Geometry check sheet. Reference: the model listing, model coordinates, mm. Face numbers are marked on the shaded views. A direction names the side the tool comes from. Coordinates: 2 decimals unless noted, no trailing zeros. Order: outer loops, then holes, each group sorted by start corner. A loop starts at its lowest first (then second) coordinate and runs counter-clockwise, first axis right, second up.
Autodesk Inventor part; units mm, degrees
ref_plane "YZ Plane" through (0, 0, 0) normal (1, 0, 0) x (0, 1, 0)
ref_plane "XZ Plane" through (0, 0, 0) normal (0, 1, 0) x (-1, 0, 0)
ref_plane "XY Plane" through (0, 0, 0) normal (0, 0, 1) x (1, 0, 0)
sketch "Skizze1" plane through (0, 0, 0) normal (0, 1, 0) x (-1, 0, 0)
  circle A0 centre (0, 0) radius 3.5
  dimension "d0" = 7
extrude "Extrusion1" add sketch "Skizze1" along normal blind 13
sketch "Skizze2" plane through (0, 13, 0) normal (0, 1, 0) x (1, 0, 0)
  circle A0 centre (0, 0) radius 2.5
  dimension "d3" = 5
extrude "Extrusion2" cut sketch "Skizze2" against normal blind 0.35
sketch "Skizze3" plane through (0, 12.65, 0) normal (0, 1, 0) x (1, 0, 0)
  line L0 (0, 0) -> (0, 2.5) construction
  circle A0 centre (0, 0) radius 2.5 construction
  circle A1 centre (-1.27, 0) radius 0.75
  circle A2 centre (1.27, 0) radius 0.75
  dimension "d6" = 1.5
  dimension "d7" = 2.54
extrude "Extrusion3" cut sketch "Skizze3" against normal through all
properties part number "Abstandhalter_13mm" material "PC/ABS-Kunststoff"
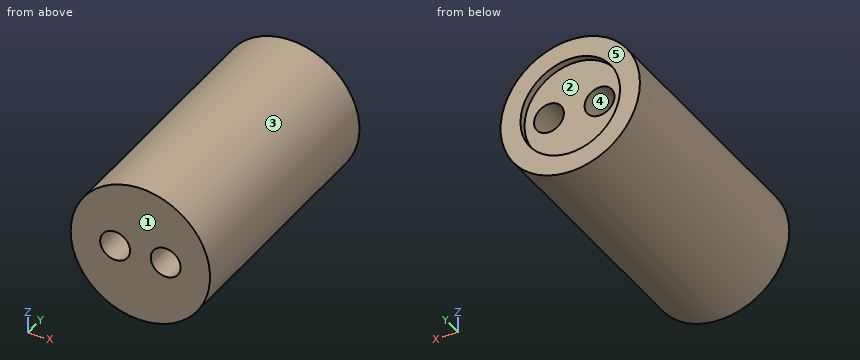
Item 1: Sectioned sample at A-A (z = 0). Record the cut outline in (x, y), and give its area (3 significant figures).
Item 2: Release check for a two-part mould opening along Z. For the marked faces 3, 4 and 5 record: pulls with the +Z half, pulls with the -Z half, needs draft (parallel to the pull), parting line crosses it, or undercut.
Item 3: Sectioned sample at C-C (x = 0.75). Record the cut outline in (y, z).
Item 4: Sectioned sample at D-D (y = 7.5). Record the cut outline in (x, z), and give its area (3 significant figures).
Item 5: Depth check by flat-ended pin: P1, Ø3, axis at x = 2, y = 3, coming from the +Z side; P2, Ø1, axis at x = -1, z = -0.5, coming from the -Y side; P3, Ø1.2, axis at x = 1.27, z = 0, coming from the +Y side; P4, Ø1.5, axis at y = 4.5, z = 2.5, coming from the +X side. Enter the tip coordinate at first touch or a pass-through.
Item 6: Sectioned sample at B-B (x = 0). Record the cut outline in (y, z), and give its area (4 significant figures).
Item 7: Tool access check on the marked faces 1 and 2. Record the directions out of +Z, -Z, +X, -X, +Y, -Y that give a thin tool (end or side, any length) a straight path to the whole face; none if there is none.
Item 8: Thickness scan on line 1 along Z through (x, y) = (0, 12.9); line 2 along Y through (x, z) = (1, 0.75); line 3 along X through (y, z) = (1, 0.5). Record the ranges inside material, lowest first.
Geometry check:
1. outline: (-3.5, 0) - (-2.02, 0) - (-2.02, 12.65) - (-2.5, 12.65) - (-2.5, 13) - (-3.5, 13) - close; (-0.52, 0) - (0.52, 0) - (0.52, 12.65) - (-0.52, 12.65) - close; (2.02, 0) - (3.5, 0) - (3.5, 13) - (2.5, 13) - (2.5, 12.65) - (2.02, 12.65) - close
1. area: 51.3 mm2
2. face 3: parting line crosses it
2. face 4: undercut
2. face 5: needs draft
3. outline: (0, -3.42) - (13, -3.42) - (13, -2.38) - (12.65, -2.38) - (12.65, -0.54) - (0, -0.54) - close; (0, 0.54) - (12.65, 0.54) - (12.65, 2.38) - (13, 2.38) - (13, 3.42) - (0, 3.42) - close
4. outline: circle Ø7 at (0, 0); hole circle Ø1.5 at (-1.27, 0); hole circle Ø1.5 at (1.27, 0)
4. area: 35.0 mm2
5. P1: stops at z = 3.46
5. P2: stops at y = 0
5. P3: passes through
5. P4: stops at x = 3.03
6. outline: (0, -3.5) - (13, -3.5) - (13, -2.5) - (12.65, -2.5) - (12.65, 2.5) - (13, 2.5) - (13, 3.5) - (0, 3.5) - close
6. area: 89.25 mm2
7. face 1: +Z, -Z, +X, -X, -Y
7. face 2: +Y
8. line 1: z = -3.5 to -2.5, 2.5 to 3.5
8. line 2: y = 0 to 12.65
8. line 3: x = -3.46 to -1.83, -0.71 to 0.71, 1.83 to 3.46
